Model file for the job. Use its own axes, mm. A direction names the side the tool comes from. Coordinates: 2 decimals unless noted, no trailing zeros. Write each loop counter-clockwise with the first axis right and the second up, starting at its lowest first coordinate (ties: lowest second). Pieces come first, ordered by that corner, then holes.
Q1. Band-saw the part on B-B, the plane y = 17. Write the cut outline in (x, z), plus the area to 3 significant figures.
Q2. Band-saw the part on C-C, the plane x = -297. Write the cut outline in (y, z).
Q3. Pull direction Y, two halves, no side cores. Call faces 3 (the flat face through (-8, -30, 20)), 4 (the flat face through (-8, -27, 20)), 5 (the flat face through (-572.5, -2, 38)): released by +Y, released by -Y, zero draft, split by the parting line, or undercut.
Q4. Drill centre lines: probe 1 along Z at (x, y) = (353, -2); probe 2 along Y at (x, z) = (-505, 25.5). Where is each one in solid material? Low to high.
Q5. Band-saw the part on A-A, the plane z = 21. Write the cut outline in (x, y).
Q6. Which spindle directions (+Z, -Z, +X, -X, +Y, -Y) get a long thin tool onto all of the face, cutting with end or side? Do faces 1 (the flat face through (-8, 27, 20)), 2 (the flat face through (-8, 0, 0)). Say none if no direction does.
from build123d import *

# Parameters (mm, degrees)
F0_W     = 1145
F0_H     = 60
F1_DEPTH = 40
F2_T     = -3


with BuildPart() as f1:
    # F0 (on Top) → F1 (new body)
    with BuildSketch(Plane.XY):
        Rectangle(F0_W, F0_H)
    extrude(amount=F1_DEPTH)

    # F2
    f2_openings = [f1.faces().sort_by_distance(p)[0] for p in [
        (-572.5, 0, 20),
        (572.5, 0, 20),
    ]]
    offset(amount=F2_T, openings=f2_openings)


solid = f1.part
Answer sheet:
1. outline: (-572.5, 0) - (572.5, 0) - (572.5, 3) - (-572.5, 3) - close; (-572.5, 37) - (572.5, 37) - (572.5, 40) - (-572.5, 40) - close
1. area: 6,870 mm2
2. outline: (-30, 0) - (30, 0) - (30, 40) - (-30, 40) - close; hole (-27, 3) - (27, 3) - (27, 37) - (-27, 37) - close
3. face 3: released by -Y
3. face 4: undercut
3. face 5: zero draft
4. probe 1: z = 0 to 3, 37 to 40
4. probe 2: y = -30 to -27, 27 to 30
5. outline: (-572.5, -30) - (572.5, -30) - (572.5, -27) - (-572.5, -27) - close; (-572.5, 27) - (572.5, 27) - (572.5, 30) - (-572.5, 30) - close
6. face 1: +X, -X
6. face 2: -Z, +X, -X, +Y, -Y
